```python
from build123d import *

# Parameters (mm, degrees)
SKETCH2_R               = 30
SKETCH2_R_2             = 18
BOSS_EXTRUDE1_DEPTH     = 27
SKETCH2_3_R             = 30
BOSS_EXTRUDE2_DEPTH     = 33
CUT_EXTRUDE1_DEPTH      = 66
CUT_EXTRUDE1_DEPTH_BACK = 66
SKETCH2_4_R             = 18


with BuildPart() as part:
    # Sketch2 → Boss-Extrude1 (new, symmetric)
    # profile 1 of 3: a face of its own
    with BuildSketch(Plane.XY):
        with BuildLine():
            ThreePointArc((0, -30), (-30, 0), (0, 30))
            Line((0, 30), (-82, 30))
            Line((-82, 30), (-82, 36))
            Line((-82, 36), (-122, 36))
            Line((-122, 36), (-122, -4))
            Line((-122, -4), (-104, -4))
            Line((-104, -4), (-44, -30))
            Line((-44, -30), (0, -30))
        make_face()
    # profile 2 of 3: a face of its own
    with BuildSketch(Plane.XY):
        Circle(SKETCH2_R)
        Circle(SKETCH2_R_2, mode=Mode.SUBTRACT)
    # profile 3 of 3: a face of its own
    with BuildSketch(Plane.XY):
        Circle(SKETCH2_R_2)
    extrude(amount=BOSS_EXTRUDE1_DEPTH, both=True)

    # Sketch2_3 → Boss-Extrude2 (add, symmetric)
    with BuildSketch(Plane.XY):
        Circle(SKETCH2_3_R)
    extrude(amount=BOSS_EXTRUDE2_DEPTH, both=True)

    # Sketch2_4 → Cut-Extrude1 (cut, two sides: drawn at the far end of the back side and taken through both)
    with BuildSketch(Plane.XY.offset(-CUT_EXTRUDE1_DEPTH_BACK)):
        Circle(SKETCH2_4_R)
    extrude(amount=CUT_EXTRUDE1_DEPTH + CUT_EXTRUDE1_DEPTH_BACK, mode=Mode.SUBTRACT)


solid = part.part
```
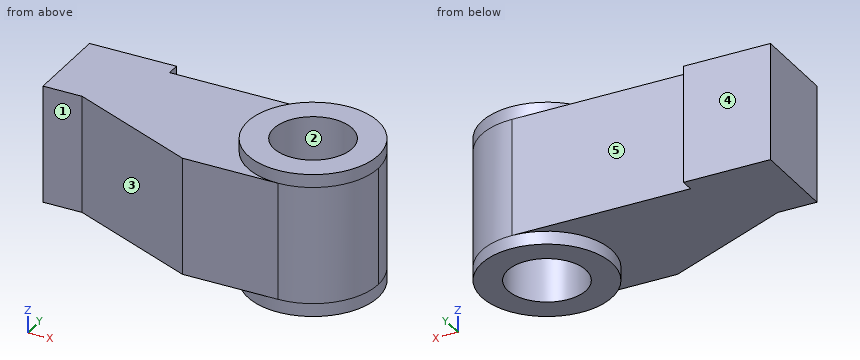
Geometry check sheet. Reference: the model listing, model coordinates, mm. Face numbers are marked on the shaded views. A direction names the side the tool comes from. Give positions to 0.01 mm unless a question says otherwise; leave off trailing zeros. Write each loop counter-clockwise with the first axis right and the second up, starting at its lowest first coordinate (ties: lowest second). Pieces come first, ordered by that corner, then holes.
1) Section check D-D, the plane y = -22.5. Record the boundary of the cut face in (x, z), and give its area (3 significant figures).
2) Release check for a two-part mould opening along X. For the marked faces 1, 2 and 3 record: pulls with the +X half, pulls with the -X half, needs draft (parallel to the pull), parting line crosses it, or undercut.
3) Gauge pin test, flat ends, axial feed: pin 1 (6 mm diameter, centred on x = -81, z = -3.5, fed in from -Y); pin 2 (14.5 mm diameter, centred on x = -115, z = -4.5, fed in from -Y); pin 3 (6 mm diameter, centred on x = -101, z = -1.5, fed in from -Y). Record the tip position at first contact, or that the pin passes through.
4) Material ranges on L1, parallel to Y at x = 0, z = 20.5; L2, parallel to X at y = 0, z = 10; L3, parallel to Z at x = -63, y = -15.5, recorded low to high.
5) Section check B-B, the plane x = -3.5. Record the boundary of the cut face in (y, z), and give its area (3 significant figures).
6) Access from +Z, -Z, +X, -X, +Y, -Y to the whole of each face (thin tool, end or side, straight path). Record for the marked faces 4 and 5.
7) Section check C-C, the plane y = 11.5. Record the boundary of the cut face in (x, z).
8) Section check A-A, the plane z = 11.5. Record the boundary of the cut face in (x, y), and give its area (3 significant figures).
Computed:
1. outline: (-61.31, -27) - (-19.84, -27) - (-19.84, -33) - (19.84, -33) - (19.84, 33) - (-19.84, 33) - (-19.84, 27) - (-61.31, 27) - close
1. area: 4,860 mm2
2. face 1: needs draft
2. face 2: undercut
2. face 3: pulls with the -X half
3. pin 1: stops at y = -15.27
3. pin 2: stops at y = -4
3. pin 3: stops at y = -6.6
4. L1: y = -30 to -18, 18 to 30
4. L2: x = -122 to -18, 18 to 30
4. L3: z = -27 to 27
5. outline: (-30, -27) - (-29.8, -27) - (-29.8, -33) - (-17.66, -33) - (-17.66, 33) - (-29.8, 33) - (-29.8, 27) - (-30, 27) - close; (17.66, -33) - (29.8, -33) - (29.8, -27) - (30, -27) - (30, 27) - (29.8, 27) - (29.8, 33) - (17.66, 33) - close
5. area: 1,620 mm2
6. face 4: +Z, -Z, +X, -X, +Y
6. face 5: +Z, -Z, +X, +Y
7. outline: (-122, -27) - (-27.71, -27) - (-27.71, -33) - (-13.85, -33) - (-13.85, 33) - (-27.71, 33) - (-27.71, 27) - (-122, 27) - close; (13.85, -33) - (27.71, -33) - (27.71, 33) - (13.85, 33) - close
8. outline: (-122, -4) - (-104, -4) - (-44, -30) - (0, -30) arc R30 ccw to (0, 30) - (-82, 30) - (-82, 36) - (-122, 36) - close; hole circle Ø36 at (0, 0)
8. area: 6,710 mm2
